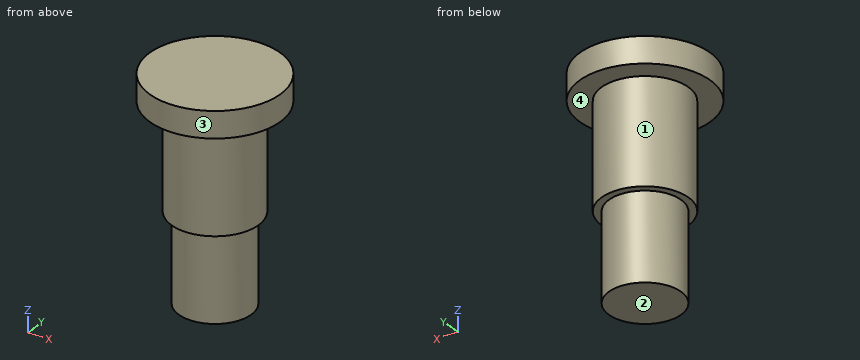
```python
from build123d import *

# Parameters (mm, degrees)
M10_START                                     = -10
SKETCH1_R                                     = 4.15
M10_ROD_ENGAGEMENT_THREAD_CORE_REPRESEN_DEPTH = 10
SKETCH2_R                                     = 5
FLOATING_SHOULDER_THROUGH_BRIDGE_DEPTH        = 12
CAPTIVE_START                                 = 12
SKETCH3_R                                     = 7.5
CAPTIVE_THRUST_HEAD_DEPTH                     = 3


with BuildPart() as part:
    # Sketch1 → M10 rod engagement, thread core represented (new body)
    with BuildSketch(Plane.XY.offset(M10_START)):
        Circle(SKETCH1_R)
    extrude(amount=M10_ROD_ENGAGEMENT_THREAD_CORE_REPRESEN_DEPTH)

    # Sketch2 → Floating shoulder through bridge (add)
    with BuildSketch(Plane.XY):
        Circle(SKETCH2_R)
    extrude(amount=FLOATING_SHOULDER_THROUGH_BRIDGE_DEPTH)

    # Sketch3 → Captive thrust head (add)
    with BuildSketch(Plane.XY.offset(CAPTIVE_START)):
        Circle(SKETCH3_R)
    extrude(amount=CAPTIVE_THRUST_HEAD_DEPTH)


solid = part.part
```
Check sheet for the modelled part. Datum: model origin and axes. Units: mm. Face numbers are marked on the shaded views. A direction names the side the tool comes from. Round coordinates to 2 decimals unless told otherwise and drop trailing zeros. Order: outer loops, then holes, each group sorted by start corner. A loop starts at its lowest first (then second) coordinate and runs counter-clockwise, first axis right, second up. Notation, with made-up numbers: (32, 49.5) - (74, 49.5) arc R32 cw to (74, 76.5) - close; hole circle Ø10 at (23, -15). An arc over 180 degrees is marked (long way). Answer as CSV lines item,"result". Start each with the question number.
1) Tool access check on the marked faces 3 and 4. Record the directions out of +Z, -Z, +X, -X, +Y, -Y that give a thin tool (end or side, any length) a straight path to the whole face; none if there is none.
2) Draft check along X on the marked faces 1 and 2. Enter one of: +X half, -X half, draft (parallel to the pull), parting line (faces both ways), or undercut.
3) Section check D-D (y = -6). Record the cut outline in (x, z).
4) Depth check by flat-ended pin: pin 1 (6 mm diameter, centred on y = -5, z = 4, fed in from -X); pin 2 (4 mm diameter, centred on y = 2.5, z = 7, fed in from -X); pin 3 (1.5 mm diameter, centred on y = -2.5, z = 2, fed in from -X). Enter the tip coordinate at first touch or a pass-through.
5) Section check C-C (z = 2.5). Record the cut outline in (x, y), then the cut area to 3 significant figures.
6) Scan lines: probe 1 along Z at (x, y) = (-3, 6.25); probe 2 along Z at (x, y) = (-4.5, 0.75); probe 3 along X at (y, z) = (3, -4). Record each from-to range of solid material in increasing order.
7) Section check A-A (x = 0). Record the cut outline in (y, z), then the cut area to 3 significant figures.
Determined:
1,face 3,"+Z, -Z"
1,face 4,"-Z"
2,face 1,"parting line"
2,face 2,"draft"
3,outline,"(-4.5, 12) - (4.5, 12) - (4.5, 15) - (-4.5, 15) - close"
4,pin 1,"x = -4.58"
4,pin 2,"x = -4.97"
4,pin 3,"x = -4.68"
5,outline,"circle Ø10 at (0, 0)"
5,area,"78.5 mm^2"
6,probe 1,"12 to 15"
6,probe 2,"0 to 15"
6,probe 3,"-2.87 to 2.87"
7,outline,"(-7.5, 12) - (-5, 12) - (-5, 0) - (-4.15, 0) - (-4.15, -10) - (4.15, -10) - (4.15, 0) - (5, 0) - (5, 12) - (7.5, 12) - (7.5, 15) - (-7.5, 15) - close"
7,area,"248 mm^2"
